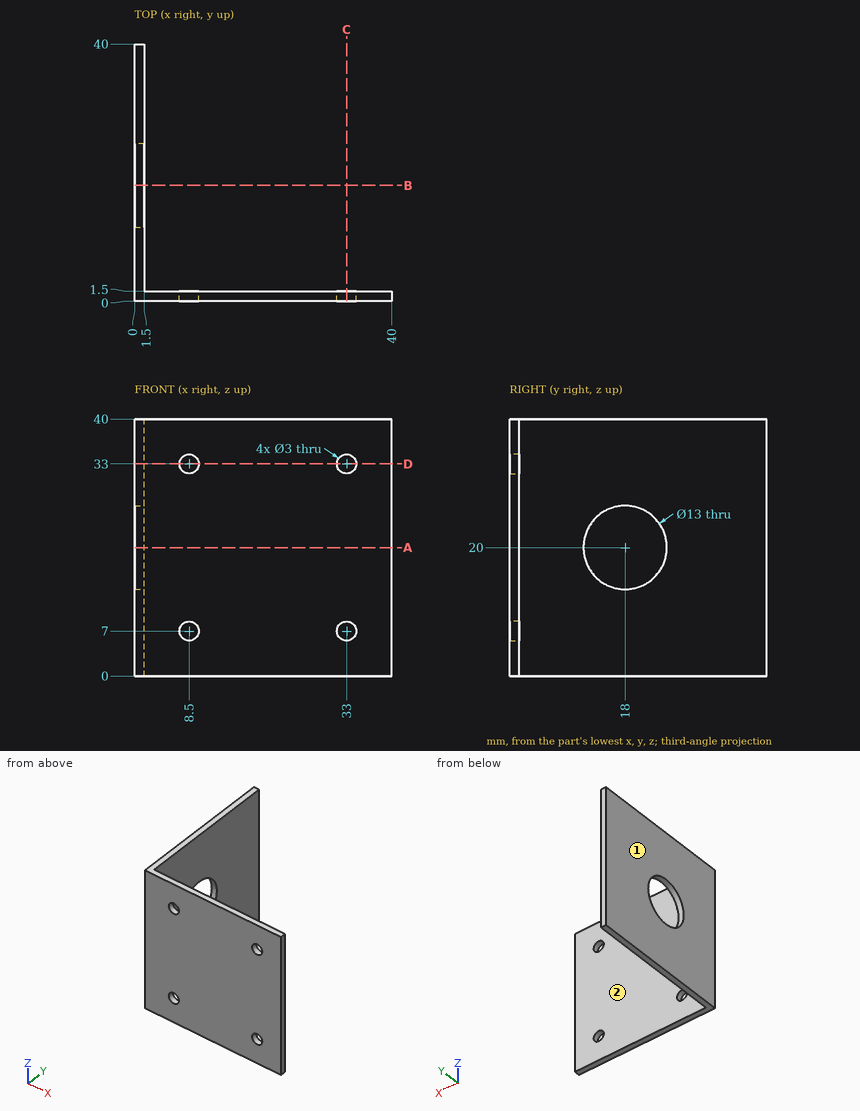
Input: dimensioned drawing with shaded views. Units: mm. Origin: part minimum x, y, z. A direction names the side the tool comes from. Give positions to 0.01 mm unless a question says otherwise; leave off trailing zeros. Loops run counter-clockwise (first coordinate to the right, second up) from the corner with the lowest first, then second, coordinate; pieces in that order, holes last. Notation, with made-up numbers: (24.25, 60.5) -> (38.25, 60.5) arc R30 cw to (38.25, 89.5) -> close; hole circle Ø6 at (9.5, 82.5). An arc over 180 degrees is marked (long way). Use a Markdown table: item, result. Add a question column.
1) Section query C-C, the plane x = 33. Return the cut outline in (y, z).
2) Section query B-B, the plane y = 18. Return the cut outline in (x, z), then the cut area to 3 significant figures.
3) Section query A-A, the plane z = 20. Return the cut outline in (x, y).
4) First-contact query: pin 1 (3 mm diameter, centred on x = 8, z = 20.5, fed in from +Y); pin 2 (11.5 mm diameter, centred on y = 28.5, z = 10.5, fed in from +X); pin 3 (1.8 mm diameter, centred on x = 33, z = 33, fed in from +Y). Flat tips, straight axial feed; report the tip coordinate or a pass-through.
5) Section query D-D, the plane z = 33. Return the cut outline in (x, y), then the cut area to 3 significant figures.
6) Reachability of the marked faces 1 and 2 from +Z, -Z, +X, -X, +Y, -Y: full face, straight path, thin tool, end or side. Return the list, or none.
7) Line query: line 1 along X through (y, z) = (0.4, 7); line 2 along X through (y, z) = (32.5, 25). Output: solid intervals per line, ascending. Write a range as [from, to].
Numbers:
| question | item | result |
|---|---|---|
| 1 | outline | (0, 0) -> (1.5, 0) -> (1.5, 5.5) -> (0, 5.5) -> close; (0, 8.5) -> (1.5, 8.5) -> (1.5, 31.5) -> (0, 31.5) -> close; (0, 34.5) -> (1.5, 34.5) -> (1.5, 40) -> (0, 40) -> close |
| 2 | outline | (0, 0) -> (1.5, 0) -> (1.5, 13.5) -> (0, 13.5) -> close; (0, 26.5) -> (1.5, 26.5) -> (1.5, 40) -> (0, 40) -> close |
| 2 | area | 40.5 mm2 |
| 3 | outline | (0, 0) -> (40, 0) -> (40, 1.5) -> (1.5, 1.5) -> (1.5, 11.5) -> (0, 11.5) -> close; (0, 24.5) -> (1.5, 24.5) -> (1.5, 40) -> (0, 40) -> close |
| 4 | pin 1 | stops at y = 1.5 |
| 4 | pin 2 | stops at x = 1.5 |
| 4 | pin 3 | passes through |
| 5 | outline | (0, 0) -> (7, 0) -> (7, 1.5) -> (1.5, 1.5) -> (1.5, 40) -> (0, 40) -> close; (10, 0) -> (31.5, 0) -> (31.5, 1.5) -> (10, 1.5) -> close; (34.5, 0) -> (40, 0) -> (40, 1.5) -> (34.5, 1.5) -> close |
| 5 | area | 109 mm2 |
| 6 | face 1 | +Z, -Z, -X, +Y, -Y |
| 6 | face 2 | +Z, -Z, +X, +Y |
| 7 | line 1 | x = [0, 7], [10, 31.5], [34.5, 40] |
| 7 | line 2 | x = [0, 1.5] |
